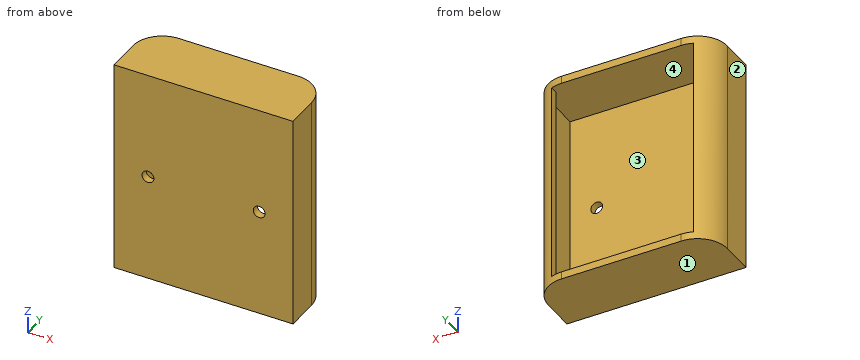
Autodesk Inventor part; units mm, degrees
ref_plane "YZ Plane" through (0, 0, 0) normal (1, 0, 0) x (0, 1, 0)
ref_plane "XZ Plane" through (0, 0, 0) normal (0, 1, 0) x (-1, 0, 0)
ref_plane "XY Plane" through (0, 0, 0) normal (0, 0, 1) x (1, 0, 0)
sketch "スケッチ1" plane through (0, 0, 0) normal (0, 1, 0) x (-1, 0, 0)
  line L0 (-24.15, -29) -> (24.15, -29)
  line L1 (24.15, -29) -> (24.15, 29)
  line L2 (24.15, 29) -> (-24.15, 29)
  line L3 (-24.15, 29) -> (-24.15, -29)
  line L4 (-24.15, -29) -> (24.15, 29) construction
  line L5 (24.15, -29) -> (-24.15, 29) construction
  point P0 (0, 0)
  dimension "d0" = 48.3
  dimension "d1" = 58
extrude "押し出し1" add sketch "スケッチ1" along normal blind 17
fillet "フィレット1" radius 8 2 edges at (24.15, 17, 0) (-24.15, 17, 0)
shell "シェル1" thickness 2 removed faces 0
sketch "スケッチ2" plane through (0, 17, 0) normal (0, 1, 0) x (1, 0, 0)
  line L0 (22.15, 27) -> (-22.15, 27)
  line L1 (19.15, -27) -> (-19.15, -27)
  line L2 (-19.15, -27) -> (-19.15, 27)
  line L3 (-19.15, 27) -> (19.15, 27)
  line L4 (19.15, 27) -> (19.15, -27)
  line L5 (19.15, -27) -> (-19.15, 27) construction
  line L6 (-19.15, -27) -> (19.15, 27) construction
  line L7 (-16.15, -29) -> (-16.15, 29)
  point P0 (0, 0)
  dimension "d8" = 3
extrude "押し出し2" cut sketch "スケッチ2" against normal blind 5
sketch "スケッチ3" plane through (-22.15, 2, 27) normal (0, 1, 0) x (1, 0, 0)
  circle A0 centre (37.15, 27) radius 1.6
  circle A1 centre (7.15, 27) radius 1.6
  line L0 (6, 54) -> (38.3, 54)
  line L1 (22.15, 54) -> (22.15, 0) construction
  line L2 (0, 0) -> (44.3, 0)
  point P0 (22.15, 27)
  dimension "d9" = 3.2
  dimension "d11" = 30
extrude "押し出し3" cut sketch "スケッチ3" against normal through all
properties part number "battery_box"
Geometry check sheet. Reference: the model listing, model coordinates, mm. Face numbers are marked on the shaded views. Give positions to 0.01 mm unless a question says otherwise; leave off trailing zeros. Write each loop counter-clockwise with the first axis right and the second up, starting at its lowest first coordinate (ties: lowest second). Pieces come first, ordered by that corner, then holes.
1) Release check for a two-part mould opening along X. For the marked faces 1, 2, 3 and 4 record: released by +X, released by -X, zero draft, split by the parting line, or undercut.
Values follow:
face 1: zero draft
face 2: released by -X
face 3: undercut
face 4: undercut
2) Go/stop test with flat-tipped pins: pin 1 Ø8 at (x, z) = (-7, -13.5) entering from -Y; pin 2 Ø4 at (x, z) = (-15, 0) entering from +Y; pin 3 Ø3 at (x, z) = (15, 0) entering from +Y; pin 4 Ø1.8 at (y, z) = (15.5, 3) entering from +X. Record where each tip stops, or that it passes through.
Values follow:
pin 1: stops at y = 0
pin 2: stops at y = 2
pin 3: passes through
pin 4: stops at x = 21.86
3) Thickness scan on line 1 (X direction, y = 0.6, z = 0); line 2 (Z direction, x = 15, y = 1.1); line 3 (Z direction, x = -9.5, y = 9.75). Record the ranges inside material, lowest first.
Values follow:
line 1: x = -24.15 to -16.6, -13.4 to 13.4, 16.6 to 24.15
line 2: z = -29 to -1.6, 1.6 to 29
line 3: z = -29 to -27, 27 to 29
4) Cross-section at B-B (x = -15). Record the boundary of the cut face in (y, z), plus the area to 3 significant figures.
Values follow:
outline: (0, -29) - (17, -29) - (17, -27) - (2, -27) - (2, -1.6) - (0, -1.6) - close; (0, 1.6) - (2, 1.6) - (2, 27) - (17, 27) - (17, 29) - (0, 29) - close
area: 170 mm2
5) Cross-section at A-A (y = 5). Record the boundary of the cut face in (x, z), plus the area to 3 significant figures.
Values follow:
outline: (-24.15, -29) - (24.15, -29) - (24.15, 29) - (-24.15, 29) - close; hole (-22.15, -27) - (22.15, -27) - (22.15, 27) - (-22.15, 27) - close
area: 409 mm2
6) Cross-section at C-C (z = 0). Record the boundary of the cut face in (x, y).
Values follow:
outline: (-24.15, 0) - (-16.6, 0) - (-16.6, 2) - (-22.15, 2) - (-22.15, 9) arc R6 cw to (-19.15, 14.2) - (-19.15, 16.42) arc R8 ccw to (-24.15, 9) - close; (-13.4, 0) - (13.4, 0) - (13.4, 2) - (-13.4, 2) - close; (16.6, 0) - (24.15, 0) - (24.15, 9) arc R8 ccw to (19.15, 16.42) - (19.15, 14.2) arc R6 cw to (22.15, 9) - (22.15, 2) - (16.6, 2) - close
7) Cross-section at D-D (x = 5.5). Record the boundary of the cut face in (y, z), plus the area to 3 significant figures.
Values follow:
outline: (0, -29) - (17, -29) - (17, -27) - (2, -27) - (2, 27) - (17, 27) - (17, 29) - (0, 29) - close
area: 176 mm2
